Check sheet for the drawn part. Datum: minimum x, y, z corner. Units: mm. Round coordinates to 2 decimals unless told otherwise and drop trailing zeros. Order: outer loops, then holes, each group sorted by start corner. A loop starts at its lowest first (then second) coordinate and runs counter-clockwise, first axis right, second up.
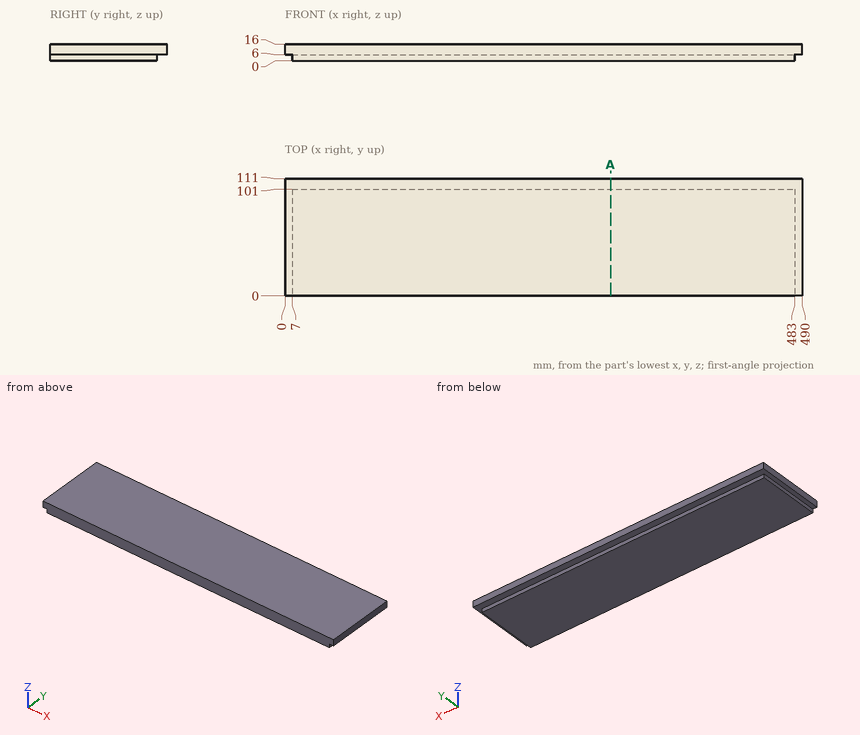
(1) Sectioned sample at A-A, the plane x = 308.5. Record the cut outline in (y, z).
Returned:
outline: (0, 0) - (101, 0) - (101, 6) - (111, 6) - (111, 16) - (0, 16) - close
(2) Material ranges on line 1 (X direction, y = 18, z = 2); line 2 (Z direction, x = 33.5, y = 103.5), recorded low to high.
Returned:
line 1: x = 7 to 483
line 2: z = 6 to 16
(3) Depth check by flat-ended pin: P1, Ø2, axis at y = 41, z = 2, coming from the -X side; P2, Ø1.8, axis at y = 32, z = 3.5, coming from the +X side; P3, Ø6.5, axis at x = 280, z = 2.5, coming from the +Y side. Enter the tip coordinate at first touch or a pass-through.
Returned:
P1: stops at x = 7
P2: stops at x = 483
P3: stops at y = 101
